from build123d import *

# Parameters (mm, degrees)
F0_W     = 30.1625
F0_H     = 57.15
F0_W_2   = 57.15
F1_DEPTH = 1.6002
F3_DEPTH = 1.6012


with BuildPart() as f1:
    # F0 (on Top) → F1 (new body)
    with BuildSketch(Plane.XY):
        Polygon((57.15, 62.70625), (57.15, 29.68625), (87.3125, 62.70625), align=None)
        Polygon((-30.1625, 62.70625), (0, 29.68625), (0, 62.70625), align=None)
        Polygon((57.15, 152.87625), (57.15, 119.85625), (87.3125, 119.85625), align=None)
        Polygon((-30.1625, 119.85625), (0, 119.85625), (0, 152.87625), align=None)
        Polygon((0, 29.68625), (0, 0), (57.15, 0), (57.15, 29.68625), (57.15, 62.70625), (0, 62.70625), align=None)
        with Locations((-15.08125, 91.28125)):
            Rectangle(F0_W, F0_H)
        with Locations((72.23125, 91.28125)):
            Rectangle(F0_W, F0_H)
        with Locations((28.575, 91.28125)):
            Rectangle(F0_W_2, F0_H)
        Polygon((0, 152.87625), (0, 119.85625), (57.15, 119.85625), (57.15, 152.87625), (57.15, 182.5625), (0, 182.5625), align=None)
    extrude(amount=F1_DEPTH)

    # F2 (on face) → F3 (cut, through all)
    with BuildSketch(Plane.XY.offset(1.6002)):
        with BuildLine():
            ThreePointArc((11.52525, 174.52975), (10.9393903391, 175.9441403391), (9.525, 176.53))
            ThreePointArc((9.525, 176.53), (8.1106096609, 175.9441403391), (7.52475, 174.52975))
            Line((7.52475, 174.52975), (7.52475, 148.71065))
            ThreePointArc((7.52475, 148.71065), (8.1106096609, 147.2962596609), (9.525, 146.7104))
            ThreePointArc((9.525, 146.7104), (10.9393903391, 147.2962596609), (11.52525, 148.71065))
            Line((11.52525, 148.71065), (11.52525, 174.52975))
        make_face()
        with BuildLine():
            ThreePointArc((49.62525, 174.52975), (49.0393903391, 175.9441403391), (47.625, 176.53))
            ThreePointArc((47.625, 176.53), (46.2106096609, 175.9441403391), (45.62475, 174.52975))
            Line((45.62475, 174.52975), (45.62475, 148.71065))
            ThreePointArc((45.62475, 148.71065), (46.2106096609, 147.2962596609), (47.625, 146.7104))
            ThreePointArc((47.625, 146.7104), (49.0393903391, 147.2962596609), (49.62525, 148.71065))
            Line((49.62525, 148.71065), (49.62525, 174.52975))
        make_face()
        with BuildLine():
            ThreePointArc((7.52475, 8.03275), (8.1106096609, 6.6183596609), (9.525, 6.0325))
            ThreePointArc((9.525, 6.0325), (10.9393903391, 6.6183596609), (11.52525, 8.03275))
            Line((11.52525, 8.03275), (11.52525, 33.85185))
            ThreePointArc((11.52525, 33.85185), (10.9393903391, 35.2662403391), (9.525, 35.8521))
            ThreePointArc((9.525, 35.8521), (8.1106096609, 35.2662403391), (7.52475, 33.85185))
            Line((7.52475, 33.85185), (7.52475, 8.03275))
        make_face()
        with BuildLine():
            ThreePointArc((45.62475, 8.03275), (46.2106096609, 6.6183596609), (47.625, 6.0325))
            ThreePointArc((47.625, 6.0325), (49.0393903391, 6.6183596609), (49.62525, 8.03275))
            Line((49.62525, 8.03275), (49.62525, 33.85185))
            ThreePointArc((49.62525, 33.85185), (49.0393903391, 35.2662403391), (47.625, 35.8521))
            ThreePointArc((47.625, 35.8521), (46.2106096609, 35.2662403391), (45.62475, 33.85185))
            Line((45.62475, 33.85185), (45.62475, 8.03275))
        make_face()
    extrude(amount=-F3_DEPTH, mode=Mode.SUBTRACT)


solid = f1.part
Input: part model. Units: mm. Frame: model coordinates. Round coordinates to 2 decimals unless told otherwise and drop trailing zeros. Write each loop counter-clockwise with the first axis right and the second up, starting at its lowest first coordinate (ties: lowest second). Pieces come first, ordered by that corner, then holes.
1) Cut plane D-D (y = 39.5). Return the cut outline in (x, z), then the cut area to 3 significant figures.
2) Contact query for a flat-ended pin moving along its axis: P1, Ø0.8, axis at y = 166.5, z = 0.5, coming from the -X side. Output: stop coordinate, or through.
3) Ray query, L1, parallel to X at y = 19, z = 1.2; L2, parallel to Y at x = 47.5, z = 0.95; L3, parallel to X at y = 30, z = 0.95. Return the intervals inside material, ascending.
4) Cut plane C-C (x = -17.5). Return the cut outline in (y, z).
5) Cut plane A-A (y = 160.5). Return the cut outline in (x, z).
6) Cut plane B-B (z = 0.9). Count the separate pieces of the cut face and the enclosed holes in it, then the cut area to 3 significant figures.
Geometry says:
1. outline: (-8.96, 0) - (66.11, 0) - (66.11, 1.6) - (-8.96, 1.6) - close
1. area: 120 mm2
2. P1: stops at x = 0
3. L1: x = 0 to 7.52, 11.53 to 45.62, 49.63 to 57.15
3. L2: y = 0 to 6.04, 35.85 to 146.71, 176.53 to 182.56
3. L3: x = -0.29 to 7.52, 11.53 to 45.62, 49.63 to 57.44
4. outline: (48.84, 0) - (133.72, 0) - (133.72, 1.6) - (48.84, 1.6) - close
5. outline: (0, 0) - (7.52, 0) - (7.52, 1.6) - (0, 1.6) - close; (11.53, 0) - (45.62, 0) - (45.62, 1.6) - (11.53, 1.6) - close; (49.63, 0) - (57.15, 0) - (57.15, 1.6) - (49.63, 1.6) - close
6. separate pieces: 1
6. enclosed holes: 4
6. area: 15,400 mm2
